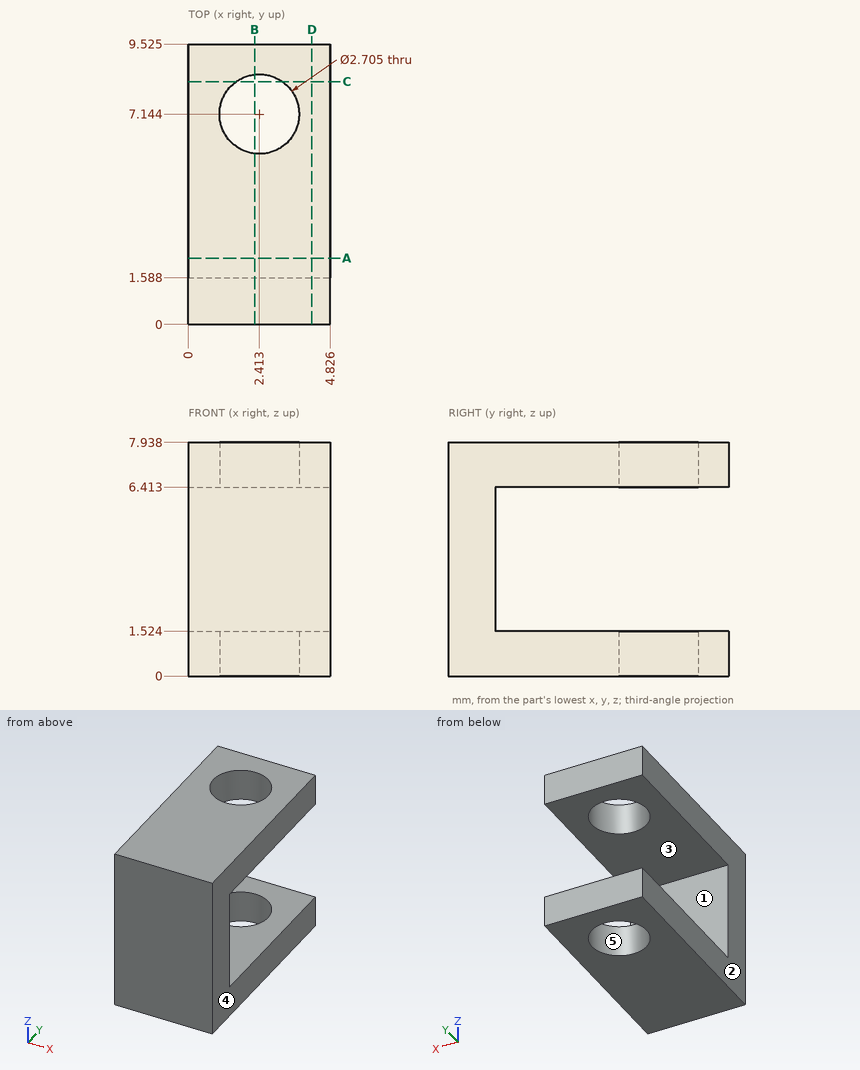
Print and shaded views of the part. All mm, measured from the part's lowest x, y and z. A direction names the side the tool comes from. Coordinates: 2 decimals unless noted, no trailing zeros. Order: outer loops, then holes, each group sorted by start corner. A loop starts at its lowest first (then second) coordinate and runs counter-clockwise, first axis right, second up. Notation, with made-up numbers: M 39,65 L 52,65 A28 ccw 52,94 Z; hole C -40,69 d11. An arc over 180 degrees is marked long. Write each question's results on one line, items separated by ' | '. Start each with the question number.
Q1. Cut at B-B (x = 2.25). List the corners of the cut face in (y, z) (1 decimal).
Q2. Drill centre lines: probe 1 along Z at (x, y) = (0.45, 5) (1 decimal); probe 2 along Y at (x, z) = (2.5, 6.5) (1 decimal); probe 3 along Y at (x, z) = (1.3, 6.25). Where is each one in solid material? Low to high. Write a range as from..to.
Q3. Cut at A-A (y = 2.25). List the corners of the cut face in (x, z) (1 decimal), then the cut area to 3 significant figures.
Q4. Cut at D-D (x = 4.2). List the corners of the cut face in (y, z) (1 decimal).
Q5. Which spindle directions (+Z, -Z, +X, -X, +Y, -Y) get a long thin tool onto all of the face, cutting with end or side? Do the marked faces 1 and 2. Say none if no direction does.
Q6. Pull direction X, two halves, no side cores. Call the marked faces 3, 4 and 5: +X half, -X half, draft (parallel to the pull), parting line (faces both ways), or undercut.
Q7. Cut at C-C (y = 8.25). List the corners of the cut face in (x, z) (1 decimal).
Found:
1) outline: M 0,0 L 5.8,0 L 5.8,1.5 L 1.6,1.5 L 1.6,6.4 L 5.8,6.4 L 5.8,7.9 L 0,7.9 Z; M 8.5,0 L 9.5,0 L 9.5,1.5 L 8.5,1.5 Z; M 8.5,6.4 L 9.5,6.4 L 9.5,7.9 L 8.5,7.9 Z
2) probe 1: 0..1.5, 6.4..7.9 | probe 2: 0..5.8, 8.5..9.5 | probe 3: 0..1.59
3) outline: M 0,0 L 4.8,0 L 4.8,1.5 L 0,1.5 Z; M 0,6.4 L 4.8,6.4 L 4.8,7.9 L 0,7.9 Z | area: 14.7 mm²
4) outline: M 0,0 L 9.5,0 L 9.5,1.5 L 1.6,1.5 L 1.6,6.4 L 9.5,6.4 L 9.5,7.9 L 0,7.9 Z
5) face 1: +X, -X, +Y | face 2: +Z, -Z, -X, +Y, -Y
6) face 3: draft | face 4: +X half | face 5: undercut
7) outline: M 0,0 L 1.6,0 L 1.6,1.5 L 0,1.5 Z; M 0,6.4 L 1.6,6.4 L 1.6,7.9 L 0,7.9 Z; M 3.2,0 L 4.8,0 L 4.8,1.5 L 3.2,1.5 Z; M 3.2,6.4 L 4.8,6.4 L 4.8,7.9 L 3.2,7.9 Z
